The model under review builds one solid part; all positions refer to its coordinate system, in mm. Face numbers are marked on the shaded views. A direction names the side the tool comes from. Coordinates: 2 decimals unless noted, no trailing zeros. Order: outer loops, then holes, each group sorted by start corner. A loop starts at its lowest first (then second) coordinate and runs counter-clockwise, first axis right, second up. Notation, with made-up numbers: M 39,32.25 L 52,32.25 A15 ccw 52,37.25 Z; hole C -30.75,33.25 d3. An arc over 180 degrees is marked long. Answer in a Markdown table with one row per item.
Autodesk Inventor part; units mm, degrees
ref_plane "YZ Plane" through (0, 0, 0) normal (1, 0, 0) x (0, 1, 0)
ref_plane "XZ Plane" through (0, 0, 0) normal (0, 1, 0) x (-1, 0, 0)
ref_plane "XY Plane" through (0, 0, 0) normal (0, 0, 1) x (1, 0, 0)
sketch "Sketch1" plane through (0, 0, 0) normal (0, 0, 1) x (1, 0, 0)
  line L0 (0, 0) -> (13.2105, 0)
  line L1 (13.2105, 0) -> (13.2105, 15.1511)
  line L2 (13.2105, 15.1511) -> (0, 15.1511)
  line L3 (0, 15.1511) -> (0, 0)
  circle A0 centre (6.6053, 9.431) radius 1.905
  dimension "d0" = 13.2105
  dimension "d1" = 15.1511
  dimension "d2" = 3.81
  dimension "d3" = 5.7201
extrude "Extrusion1" add sketch "Sketch1" along normal blind 1.1989
sketch "Sketch2" plane through (0, 0, 0) normal (0, -1, 0) x (1, 0, 0)
  line L0 (0, 0) -> (13.2105, 0)
  line L1 (0, 1.1989) -> (1.1989, 1.1989)
  line L2 (1.1989, 1.1989) -> (1.1989, 0)
  line L3 (1.1989, 0) -> (0, 0)
  line L4 (0, 0) -> (0, 1.1989)
  line L5 (13.2105, 1.1989) -> (12.0117, 1.1989)
  line L6 (12.0117, 1.1989) -> (12.0117, 0)
  line L7 (12.0117, 0) -> (13.2105, 0)
  line L8 (13.2105, 0) -> (13.2105, 1.1989)
  dimension "d6" = 1.1989
  dimension "d7" = 1.1989
extrude "Extrusion2" add sketch "Sketch2" along normal blind 3.8989
sketch "Sketch3" plane through (0, 0, 1.1989) normal (0, 0, 1) x (1, 0, 0)
  line L0 (13.2105, -3.8989) -> (12.0117, -3.8989)
  line L1 (12.0117, -3.8989) -> (12.0117, 15.1511)
  line L2 (12.0117, 15.1511) -> (13.2105, 15.1511)
  line L3 (13.2105, 15.1511) -> (13.2105, -3.8989)
  line L4 (0, -3.8989) -> (1.1989, -3.8989)
  line L5 (1.1989, -3.8989) -> (1.1989, 15.1511)
  line L6 (1.1989, 15.1511) -> (0, 15.1511)
  line L7 (0, 15.1511) -> (0, -3.8989)
  point P0 (0, 0)
extrude "Extrusion3" add sketch "Sketch3" along normal blind 8.3312
sketch "Sketch4" plane through (13.2105, -3.8989, 0) normal (1, 0, 0) x (0, 0, -1)
  line L0 (-9.5301, 19.05) -> (-9.5301, 0)
  line L1 (0, 19.05) -> (-9.5301, 19.05)
  line L2 (0, 19.05) -> (0, 0)
  line L3 (-9.5301, 16.5506) -> (-4.0005, 16.5506)
  line L4 (-4.0005, 16.5506) -> (-4.0005, 14.8996)
  line L5 (-4.0005, 14.8996) -> (-9.5301, 14.8996)
  line L6 (-9.5301, 14.8996) -> (-9.5301, 16.5506)
  line L7 (-9.5301, 12.4003) -> (-4.0005, 12.4003)
  line L8 (-4.0005, 12.4003) -> (-4.0005, 10.7493)
  line L9 (-4.0005, 10.7493) -> (-9.5301, 10.7493)
  line L10 (-9.5301, 10.7493) -> (-9.5301, 12.4003)
  line L11 (-9.5301, 8.2499) -> (-4.0005, 8.2499)
  line L12 (-4.0005, 8.2499) -> (-4.0005, 6.5989)
  line L13 (-4.0005, 6.5989) -> (-9.5301, 6.5989)
  line L14 (-9.5301, 6.5989) -> (-9.5301, 8.2499)
  line L15 (-9.5301, 4.097) -> (-4.0005, 4.097)
  line L16 (-4.0005, 4.097) -> (-4.0005, 2.446)
  line L17 (-4.0005, 2.446) -> (-9.5301, 2.446)
  line L18 (-9.5301, 2.446) -> (-9.5301, 4.097)
  point P0 (0, 3.8989)
  point P1 (-9.5301, 2.446)
  point P2 (-4.0005, 19.05)
  dimension "d12" = 2.4994
  dimension "d13" = 1.651
  dimension "d14" = 2.4994
  dimension "d15" = 1.651
  dimension "d16" = 2.4994
  dimension "d17" = 1.651
  dimension "d18" = 2.5019
  dimension "d19" = 1.651
  dimension "d20" = 4.0005
extrude "Extrusion4" cut sketch "Sketch4" against normal blind 25.4
fillet "Fillet1" radius 0.8255 16 edges at (12.6111, 11.0007, 4.0005) (12.6111, 6.8504, 4.0005) (12.6111, 2.7, 4.0005) (0.5994, -1.4529, 4.0005) (12.6111, -1.4529, 4.0005) (0.5994, 11.0007, 4.0005) (0.5994, 6.8504, 4.0005) (0.5994, 2.7, 4.0005) (12.6111, 12.6517, 4.0005) (12.6111, 8.5014, 4.0005) (12.6111, 4.351, 4.0005) (12.6111, 0.1981, 4.0005) (0.5994, 12.6517, 4.0005) (0.5994, 8.5014, 4.0005) (0.5994, 4.351, 4.0005) (0.5994, 0.1981, 4.0005)
fillet "Fillet2" radius 0.8255 2 edges at (13.2105, 5.6261, 0) (0, 5.6261, 0)
properties part number "TO-220 Heatsink"
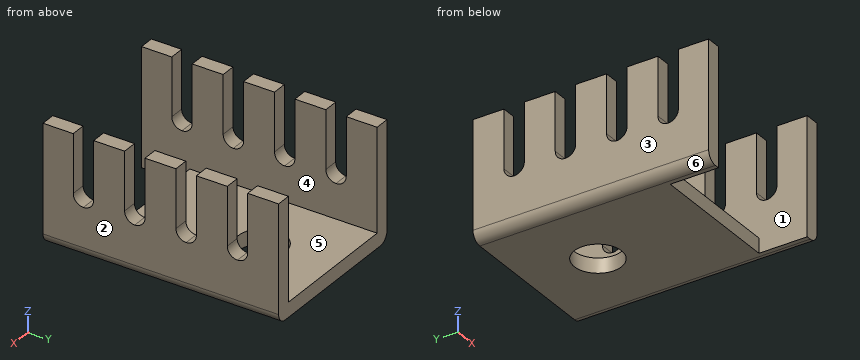
(1) Take a section at A-A (z = 2). Write out the cut boundary in (x, y).
Report:
| item | result |
|---|---|
| outline | M 0,-3.9 L 1.2,-3.9 L 1.2,15.15 L 0,15.15 Z; M 12.01,-3.9 L 13.21,-3.9 L 13.21,15.15 L 12.01,15.15 Z |
(2) The part is to be moulded in two halves that separate along X. For the marked faces 1, 2, 3 and 4, say which applies: +X half, -X half, draft (parallel to the pull), parting line (faces both ways), or undercut.
Report:
| item | result |
|---|---|
| face 1 | undercut |
| face 2 | +X half |
| face 3 | -X half |
| face 4 | undercut |
(3) Take a section at D-D (z = 5.25). State how many separate pieces and enclosed holes the cut face has, then the cut area to 3 significant figures.
Report:
| item | result |
|---|---|
| separate pieces | 10 |
| enclosed holes | 0 |
| area | 29.8 mm^2 |
(4) To check wall thickness, follow line 1 (Y direction, x = 0.75, z = 8.75); line 2 (X direction, y = 14.75, z = 2.75); line 3 (Z direction, x = 5.25, y = 11). State the ranges of each line that lie inside material, in increasing order. Write a range as [from, to].
Report:
| item | result |
|---|---|
| line 1 | [-3.9, -1.45], [0.2, 2.7], [4.35, 6.85], [8.5, 11], [12.65, 15.15] |
| line 2 | [0, 1.2], [12.01, 13.21] |
| line 3 | [0, 1.2] |
(5) Machinability: for the marked faces 5 and 6, which of the approach directions +Z, -Z, +X, -X, +Y, -Y give a long, thin tool a straight path to every point of the face, cutting with its end or side? Answer none if there is none.
Report:
| item | result |
|---|---|
| face 5 | +Z, +Y, -Y |
| face 6 | -Z, -X, +Y, -Y |
(6) Take a section at C-C (x = 5). Write out the cut boundary in (y, z).
Report:
| item | result |
|---|---|
| outline | M 0,0 L 8.41,0 L 8.41,1.2 L 0,1.2 Z; M 10.46,0 L 15.15,0 L 15.15,1.2 L 10.46,1.2 Z |
(7) Insertion check: P1, Ø4.5, axis at x = 6.61, y = 9.43, coming from the -Z side; P2, Ø1.3, axis at x = 4.5, z = 0.5, coming from the -Y side. Each pin has a flat end and moves straight along its axis. Give the tip position at first contact, or say it passes through.
Report:
| item | result |
|---|---|
| P1 | z = 0 |
| P2 | y = 0 |
